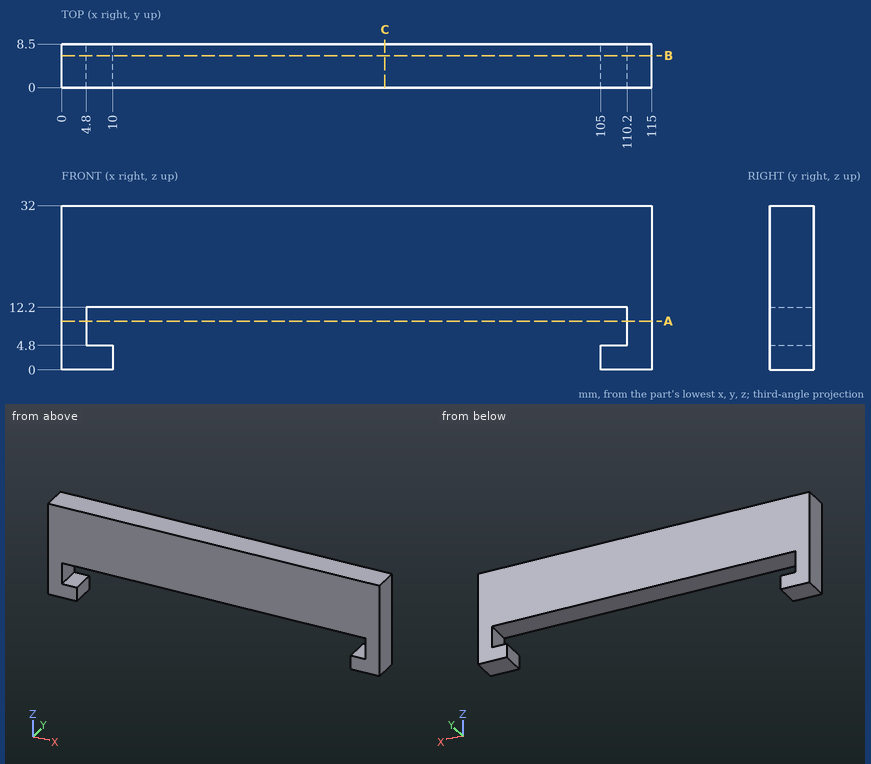
Answer from the drawing. Dimensions are ordinates in mm from the lowest x, y and z of the part. Give positions to 0.01 mm unless a question says otherwise; leave off trailing zeros. Write each loop counter-clockwise with the first axis right and the second up, starting at its lowest first coordinate (ties: lowest second). Pieces come first, ordered by that corner, then holes.
1) Section A-A (z = 9.5) is taken. Write down the section's boundary in (x, y).
2) Given P1, Ø5, axis at x = 44.5, y = 4, coming from the -Z side, flat-ended and moving along its own axis, determine where the tip first touches the part or whether it passes through.
3) Section B-B (y = 6.25) is taken. Write down the section's boundary in (x, z).
4) Section C-C (x = 63) is taken. Write down the section's boundary in (y, z).
5) Find the intervals of material crossed by L1, parallel to X at y = 8, z = 9; L2, parallel to Z at x = 52, y = 3.25, in increasing order.
Response:
1. outline: (0, 0) - (4.8, 0) - (4.8, 8.5) - (0, 8.5) - close; (110.2, 0) - (115, 0) - (115, 8.5) - (110.2, 8.5) - close
2. P1: stops at z = 12.2
3. outline: (0, 0) - (10, 0) - (10, 4.8) - (4.8, 4.8) - (4.8, 12.2) - (110.2, 12.2) - (110.2, 4.8) - (105, 4.8) - (105, 0) - (115, 0) - (115, 32) - (0, 32) - close
4. outline: (0, 12.2) - (8.5, 12.2) - (8.5, 32) - (0, 32) - close
5. L1: x = 0 to 4.8, 110.2 to 115
5. L2: z = 12.2 to 32
